from build123d import *

# Parameters (mm, degrees)
SKETCH2_W          = 558.8
SKETCH2_H          = 396.08125
EXTRUDE1_DEPTH     = 17.78
SKETCH3_R          = 15.08125
SKETCH3_R_2        = 3.4925
SKETCH3_R_3        = 1.5875
SKETCH3_W          = 308.0004
SKETCH3_H          = 261.9629
CUT_EXTRUDE1_DEPTH = 17.78
CUT_EXTRUDE2_DEPTH = 5.08
CUT_EXTRUDE4_DEPTH = 396.08125
FILLET1_R          = 20.6502


with BuildPart() as part:
    # Sketch2 → Extrude1 (new body)
    with BuildSketch(Plane.XY):
        with Locations((11975.041666666, -5854.303125)):
            Rectangle(SKETCH2_W, SKETCH2_H)
    extrude(amount=-EXTRUDE1_DEPTH)

    # Sketch3 → Cut-Extrude1 (cut)
    with BuildSketch(Plane.XY):
        with Locations((12197.291666666, -5761.0375)):
            Circle(SKETCH3_R)
        with Locations((12138.554166666, -5833.26875)):
            Circle(SKETCH3_R_2)
        with Locations((12196.974166666, -5865.01875)):
            Circle(SKETCH3_R_3)
        with Locations((12196.974166666, -5922.16875)):
            Circle(SKETCH3_R_3)
        with Locations((12196.974166666, -5979.31875)):
            Circle(SKETCH3_R_3)
        with Locations((12140.141666666, -6037.10375)):
            Circle(SKETCH3_R_3)
        with Locations((11975.041666666, -6037.10375)):
            Circle(SKETCH3_R_3)
        with Locations((11809.941666666, -6037.10375)):
            Circle(SKETCH3_R_3)
        with Locations((11753.109166666, -5979.31875)):
            Circle(SKETCH3_R_3)
        with Locations((11753.109166666, -5922.16875)):
            Circle(SKETCH3_R_3)
        with Locations((11753.109166666, -5865.01875)):
            Circle(SKETCH3_R_3)
        with Locations((11811.529166666, -5833.26875)):
            Circle(SKETCH3_R_2)
        with Locations((11975.041666666, -5973.7625)):
            Circle(SKETCH3_R_2)
        with Locations((11975.041666666, -5692.775)):
            Circle(SKETCH3_R_2)
        with Locations((11975.041666666, -5833.26875)):
            Rectangle(SKETCH3_W, SKETCH3_H)
        with BuildLine():
            Line((11734.654409808, -5693.754968556), (11739.23011943, -5693.754968556))
            ThreePointArc((11739.23011943, -5693.754968556), (11748.029166666, -5687.976468556), (11756.828213901, -5693.754968556))
            Line((11756.828213901, -5693.754968556), (11761.386355753, -5693.754968556))
            ThreePointArc((11761.386355753, -5693.754968556), (11767.531113043, -5692.357368906), (11771.079666666, -5697.564968556))
            ThreePointArc((11771.079666666, -5697.564968556), (11767.531113043, -5702.772568206), (11761.386355753, -5701.374968556))
            Line((11761.386355753, -5701.374968556), (11756.828213901, -5701.374968556))
            ThreePointArc((11756.828213901, -5701.374968556), (11754.760305425, -5704.393665595), (11751.712166666, -5706.417925308))
            Line((11751.712166666, -5706.417925308), (11751.712166666, -5721.30243896))
            ThreePointArc((11751.712166666, -5721.30243896), (11748.029166666, -5731.092968556), (11744.346166666, -5721.30243896))
            Line((11744.346166666, -5721.30243896), (11744.346166666, -5706.417925308))
            ThreePointArc((11744.346166666, -5706.417925308), (11741.298027907, -5704.393665595), (11739.23011943, -5701.374968556))
            Line((11739.23011943, -5701.374968556), (11734.654409809, -5701.374968556))
            ThreePointArc((11734.654409809, -5701.374968556), (11724.978666666, -5697.564968556), (11734.654409808, -5693.754968556))
        make_face()
    extrude(amount=-CUT_EXTRUDE1_DEPTH, mode=Mode.SUBTRACT)

    # Sketch4 → Cut-Extrude2 (cut)
    with BuildSketch(Plane.XY):
        Polygon((11975.041666666, -6028.21375), (11695.641666666, -6028.21375), (11695.641666666, -6045.99375), (12254.441666666, -6045.99375), (12254.441666666, -6028.21375), align=None)
    extrude(amount=-CUT_EXTRUDE2_DEPTH, mode=Mode.SUBTRACT)

    # Sketch7 → Cut-Extrude4 (cut)
    with BuildSketch(Plane.XZ.offset(6052.34375)):
        Polygon((11701.991666666, -11.43), (11701.991666666, 0), (11695.641666666, 0), (11695.641666666, -17.78), align=None)
        Polygon((12248.091666666, -11.43), (12254.441666666, -17.78), (12254.441666666, 0), (12248.091666666, 0), align=None)
    extrude(amount=-CUT_EXTRUDE4_DEPTH, mode=Mode.SUBTRACT)

    # Fillet1
    fillet1_edges = [part.edges().sort_by_distance(p)[0] for p in [
        (11821.041466666, -5964.2502, -8.89),
        (11821.041466666, -5702.2873, -8.89),
        (12129.041866666, -5702.2873, -8.89),
        (12129.041866666, -5964.2502, -8.89),
    ]]
    fillet(fillet1_edges, radius=FILLET1_R)


solid = part.part
For this review, take the finished solid that the model builds, in its own axes (mm). A direction names the side the tool comes from. Round coordinates to 2 decimals unless told otherwise and drop trailing zeros. Loops run counter-clockwise (first coordinate to the right, second up) from the corner with the lowest first, then second, coordinate; pieces in that order, holes last. Notation, with made-up numbers: (-7.5, 18) - (40.5, 18) arc R35 cw to (40.5, 55) - close; hole circle Ø10 at (-10, 17.25). An arc over 180 degrees is marked (long way). Use one line per item in the form item = value.
1) Clearance check with flat-ended pins moving along their axes: P1, Ø3, axis at y = -5710.5, z = -10, coming from the +X side; P2, Ø5, axis at x = 12140.14, y = -6037.1, coming from the +Z side; P3, Ø5, axis at y = -5998, z = -11.5, coming from the -X side. State where each tip first meets the part, or that it passes through.
Solutions:
P1 = 12248.16
P2 = -5.08
P3 = 11699.42
2) We need section C-C on y = -5993. Write out the cut boundary in (x, z).
Solutions:
outline = (11695.64, -17.78) - (12254.44, -17.78) - (12248.09, -11.43) - (12248.09, 0) - (11701.99, 0) - (11701.99, -11.43) - close
3) Tool access review of faces 1 (the face through (12129.042, -5835, -9)), 2 (the face through (12248.092, -5857, -6)), 3 (the face through (11701.992, -5857, -6)), 4 (the face through (11971, -6037, -5.08)): name each direction out of +Z, -Z, +X, -X, +Y, -Y from which nothing blocks a thin tool from reaching the whole face with its end or side.
Solutions:
face_1 = +Z, -Z
face_2 = +Z, +X, +Y, -Y
face_3 = +Z, -X, +Y, -Y
face_4 = +Z, +X, -X
4) Mouldability with a two-part tool opening along Y and no side actions: class faces 5 (the face through (11971, -5984, -17.78)), 6 (the face through (11971, -5656.263, -9)), 7 (the face through (11744.346, -5714, -9)) as pulls with the +Y half, pulls with the -Y half, needs draft (parallel to the pull), parting line crosses it, or undercut.
Solutions:
face_5 = needs draft
face_6 = pulls with the +Y half
face_7 = undercut
5) We need section A-A on x = 12007. Write out the cut boundary in (y, z).
Solutions:
outline = (-6052.34, -17.78) - (-5964.25, -17.78) - (-5964.25, 0) - (-6028.21, 0) - (-6028.21, -5.08) - (-6045.99, -5.08) - (-6045.99, 0) - (-6052.34, 0) - close; (-5702.29, -17.78) - (-5656.26, -17.78) - (-5656.26, 0) - (-5702.29, 0) - close
6) Wall thickness on probe 1 along Y at (x, z) = (11880, -2); probe 2 along Y at (x, z) = (11908, -7.25); probe 3 along Y at (x, z) = (12139.5, -7.25): over which ranges is each line inside the solid? List them lowest first.
Solutions:
probe_1 = -6052.34 to -6045.99, -6028.21 to -5964.25, -5702.29 to -5656.26
probe_2 = -6052.34 to -5964.25, -5702.29 to -5656.26
probe_3 = -6052.34 to -6038.56, -6035.65 to -5836.63, -5829.91 to -5656.26
7) We need section B-B on y = -5887. Write out the cut boundary in (x, z), then the cut area to 3 significant figures.
Solutions:
outline = (11695.64, -17.78) - (11821.04, -17.78) - (11821.04, 0) - (11701.99, 0) - (11701.99, -11.43) - close; (12129.04, -17.78) - (12254.44, -17.78) - (12248.09, -11.43) - (12248.09, 0) - (12129.04, 0) - close
area = 4,270 mm2
